Work out the finished part from the listing and answer in its coordinate system (mm). A direction names the side the tool comes from. Round coordinates to 2 decimals unless told otherwise and drop trailing zeros. Loops run counter-clockwise (first coordinate to the right, second up) from the corner with the lowest first, then second, coordinate; pieces in that order, holes last. Notation, with made-up numbers: (19.25, -19.75) -> (60.25, -19.75) arc R9 ccw to (60.25, -6.75) -> close; hole circle Ø2 at (21.5, 78.25). An arc over 180 degrees is marked (long way). Use one line per item in the form item = value.
```python
from build123d import *

# Parameters (mm, degrees)
F1_DEPTH = 12.5
F2_R     = 10
F3_DEPTH = 30
F4_SIZE  = 2
F5_W     = 10
F5_H     = 32.5
F6_DEPTH = 25


# Not quite as in the source:
# - a pattern or mirror of a feature is missing from the dataset's text; its kind, count and spacing are read off the source's solid


with BuildPart() as f1:
    # F0 (on Top) → F1 (new body, symmetric)
    with BuildSketch(Plane.XY):
        Polygon((-15, -15), (-12, -40), (12, -40), (15, -15), (15, 15), (12, 40), (-12, 40), (-15, 15), align=None)
    extrude(amount=F1_DEPTH, both=True)

    # F2 (on face) → F3 (join)
    with BuildSketch(Plane.XZ.offset(40)):
        Circle(F2_R)
    f3 = extrude(amount=F3_DEPTH)

    # F3_copies: F3 across plane
    add(f3.mirror(Plane.ZX))

    # F4
    f4_edges = [f1.edges().sort_by_distance(p)[0] for p in [
        (-10, -70, 0),
        (-10, 70, 0),
    ]]
    chamfer(f4_edges, length=F4_SIZE)

    # F5 (on face) → F6 (cut)
    with BuildSketch(Plane.XY.offset(12.5)):
        Rectangle(F5_W, F5_H)
    extrude(amount=-F6_DEPTH, mode=Mode.SUBTRACT)


solid = f1.part
```
(1) For faces 1 (the flat face through (-13.52, -27.33, 0.18)), 2 (the flat face through (-6, -40, 9)), 3 (the cylindrical face through (-2.17, 53.8, -9.76)), 4 (the flat face through (0, 70, 0)), 5 (the flat face through (5, 0, 0)), determine the directions among +Z, -Z, +X, -X, +Y, -Y from which every point of the face is accessible in a straight line to the end or side of a thin tool.
Completed:
face_1 = +Z, -Z, -X, -Y
face_2 = -Y
face_3 = +Y
face_4 = +Z, -Z, +X, -X, +Y
face_5 = +Z, -Z
(2) For a pull along X with two mould halves and no side action, classify faces 6 (the flat face through (-13.48, 27.67, 0.18)), 7 (the flat face through (0, 16.25, 0)), 8 (the flat face through (0, -70, 0)) as +X half, -X half, draft (parallel to the pull), parting line (faces both ways), or undercut.
Completed:
face_6 = -X half
face_7 = undercut
face_8 = draft
(3) Find section D-D, the plane y = -26. Write down the section's boundary in (x, z).
Completed:
outline = (-13.68, -12.5) -> (13.68, -12.5) -> (13.68, 12.5) -> (-13.68, 12.5) -> close
(4) Find section C-C, the plane z = 0. Write down the section's boundary in (x, y), then the cut area to 3 significant figures.
Completed:
outline = (-15, -15) -> (-12, -40) -> (-10, -40) -> (-10, -68) -> (-8, -70) -> (8, -70) -> (10, -68) -> (10, -40) -> (12, -40) -> (15, -15) -> (15, 15) -> (12, 40) -> (10, 40) -> (10, 68) -> (8, 70) -> (-8, 70) -> (-10, 68) -> (-10, 40) -> (-12, 40) -> (-15, 15) -> close; hole (-5, -16.25) -> (5, -16.25) -> (5, 16.25) -> (-5, 16.25) -> close
area = 3,120 mm2
(5) Find section B-B, the plane y = 8. Write down the section's boundary in (x, z).
Completed:
outline = (-15, -12.5) -> (-5, -12.5) -> (-5, 12.5) -> (-15, 12.5) -> close; (5, -12.5) -> (15, -12.5) -> (15, 12.5) -> (5, 12.5) -> close
(6) Find section A-A, the plane x = 0. Write down the section's boundary in (y, z).
Completed:
outline = (-70, -8) -> (-68, -10) -> (-40, -10) -> (-40, -12.5) -> (-16.25, -12.5) -> (-16.25, 12.5) -> (-40, 12.5) -> (-40, 10) -> (-68, 10) -> (-70, 8) -> close; (16.25, -12.5) -> (40, -12.5) -> (40, -10) -> (68, -10) -> (70, -8) -> (70, 8) -> (68, 10) -> (40, 10) -> (40, 12.5) -> (16.25, 12.5) -> close
(7) Consider L1, parallel to Y at x = -3, z = 3.25; L2, parallel to X at y = 14.5, z = 3.5; L3, parallel to X at y = -56.5, z = -6. Determine where each line is inside the solid, lowest interval first.
Completed:
L1 = -70 to -16.25, 16.25 to 70
L2 = -15 to -5, 5 to 15
L3 = -8 to 8
(8) Given P1, Ø8, axis at x = 10, z = 7, coming from the -Y side; P2, Ø2, axis at x = -9, z = 7, coming from the +Y side; P3, Ø3, axis at x = -6.5, y = 53, coming from the -Z side, each flat-ended and moving along its own axis, determine where each tip first touches the part or whether it passes through.
Completed:
P1 = -69.79
P2 = 40
P3 = -8.66
